from build123d import *

# Parameters (mm, degrees)
BOSS_EXTRUDE1_DEPTH      = 50
FILLET2_R                = 20
SKETCH6_R                = 1.5
CUT_EXTRUDE2_DEPTH       = 28.4
CUT_EXTRUDE3_DEPTH       = 136.4
CUT_EXTRUDE4_DEPTH       = 116.893533958
CUT_EXTRUDE4_DEPTH_BACK  = 26.4
BOSS_EXTRUDE2_DEPTH      = 21.9
BOSS_EXTRUDE3_DEPTH      = 12.1
BOSS_EXTRUDE4_DEPTH      = 7.5
CUT_EXTRUDE5_START       = 12.1
CUT_EXTRUDE5_OUTLINE_R   = 2.25
CUT_EXTRUDE5_DEPTH       = 21.9
CUT_EXTRUDE5_START_2     = -7.5
CUT_EXTRUDE5_2_OUTLINE_R = 4
CUT_EXTRUDE5_2_DEPTH     = 7.5


# Read off the part's stored shape, not the designer's step: Cut-Extrude5
with BuildPart() as part:
    # Sketch1 → Boss-Extrude1 (new body)
    with BuildSketch(Plane(origin=(0, 0, 0), x_dir=(1, 0, 0), z_dir=(0, 1, 0))):
        with BuildLine():
            Line((-56.375697839, 54.197981352), (-56.375697839, 10.497981352))
            ThreePointArc((-56.375697839, 10.497981352), (-53.44676565, 3.42691354), (-46.375697839, 0.497981352))
            Line((-46.375697839, 0.497981352), (16.224302161, 0.497981352))
            ThreePointArc((16.224302161, 0.497981352), (23.295369973, 3.42691354), (26.224302161, 10.497981352))
            Line((26.224302161, 10.497981352), (26.224302161, 64.097981352))
            Line((26.224302161, 64.097981352), (19.224302161, 64.097981352))
            Line((19.224302161, 64.097981352), (19.224302161, 10.497981352))
            ThreePointArc((19.224302161, 10.497981352), (18.345622505, 8.376661008), (16.224302161, 7.497981352))
            Line((16.224302161, 7.497981352), (-46.375697839, 7.497981352))
            ThreePointArc((-46.375697839, 7.497981352), (-48.497018182, 8.376661008), (-49.375697839, 10.497981352))
            Line((-49.375697839, 10.497981352), (-49.375697839, 54.197981352))
            Line((-49.375697839, 54.197981352), (-56.375697839, 54.197981352))
        make_face()
    extrude(amount=BOSS_EXTRUDE1_DEPTH)

    # Fillet2
    fillet2_edges = [part.edges().sort_by_distance(p)[0] for p in [
        (22.724302161, 0, -64.097981352),
        (-52.875697839, 0, -54.197981352),
        (22.724302161, 50, -64.097981352),
        (-52.875697839, 50, -54.197981352),
    ]]
    fillet(fillet2_edges, radius=FILLET2_R)

    # Sketch6 → Cut-Extrude2 (cut)
    with BuildSketch(Plane(origin=(26.224302161, 0, 0), x_dir=(0, 0, -1), z_dir=(1, 0, 0))):
        with BuildLine():
            ThreePointArc((34.097981352, 25), (38.097981352, 21), (42.097981352, 25))
            Line((42.097981352, 25), (34.097981352, 25))
        make_face()
        with BuildLine():
            Line((34.097981352, 25), (42.097981352, 25))
            ThreePointArc((42.097981352, 25), (38.097981352, 29), (34.097981352, 25))
        make_face()
        with BuildLine():
            ThreePointArc((31.836343923, 25), (38.097981352, 18.738362572), (44.35961878, 25))
            Line((44.35961878, 25), (42.097981352, 25))
            ThreePointArc((42.097981352, 25), (38.097981352, 21), (34.097981352, 25))
            Line((34.097981352, 25), (31.836343923, 25))
        make_face()
        with BuildLine():
            Line((42.097981352, 25), (44.35961878, 25))
            ThreePointArc((44.35961878, 25), (38.097981352, 31.261637428), (31.836343923, 25))
            Line((31.836343923, 25), (34.097981352, 25))
            ThreePointArc((34.097981352, 25), (38.097981352, 29), (42.097981352, 25))
        make_face()
        with Locations((30.390517437, 32.707463915)):
            Circle(SKETCH6_R)
        with Locations((26.876196734, 36.221784617)):
            Circle(SKETCH6_R)
        with Locations((23.354804964, 39.743176388)):
            Circle(SKETCH6_R)
        with Locations((19.854626397, 43.243354955)):
            Circle(SKETCH6_R)
        with Locations((44.108388992, 31.01040764)):
            Circle(SKETCH6_R)
        with Locations((47.643922898, 34.545941546)):
            Circle(SKETCH6_R)
        with Locations((51.179456803, 38.081475452)):
            Circle(SKETCH6_R)
        with Locations((54.714990709, 41.617009358)):
            Circle(SKETCH6_R)
        with Locations((45.805445266, 17.292536085)):
            Circle(SKETCH6_R)
        with Locations((49.319765969, 13.778215383)):
            Circle(SKETCH6_R)
        with Locations((52.841157739, 10.256823612)):
            Circle(SKETCH6_R)
        with Locations((56.341336306, 6.756645045)):
            Circle(SKETCH6_R)
        with Locations((32.087573711, 18.98959236)):
            Circle(SKETCH6_R)
        with Locations((28.552039805, 15.454058454)):
            Circle(SKETCH6_R)
        with Locations((25.0165059, 11.918524548)):
            Circle(SKETCH6_R)
        with Locations((21.480971994, 8.382990642)):
            Circle(SKETCH6_R)
    extrude(amount=-CUT_EXTRUDE2_DEPTH, mode=Mode.SUBTRACT)

    # Sketch6<3> → Cut-Extrude3 (cut)
    with BuildSketch(Plane(origin=(26.224302161, 0, 0), x_dir=(0, 0, -1), z_dir=(1, 0, 0))):
        with BuildLine():
            ThreePointArc((34.097981352, 25), (38.097981352, 21), (42.097981352, 25))
            Line((42.097981352, 25), (34.097981352, 25))
        make_face()
        with BuildLine():
            Line((34.097981352, 25), (42.097981352, 25))
            ThreePointArc((42.097981352, 25), (38.097981352, 29), (34.097981352, 25))
        make_face()
    extrude(amount=-CUT_EXTRUDE3_DEPTH, mode=Mode.SUBTRACT)

    # Sketch7 → Cut-Extrude4 (cut, two sides: drawn at the far end of the back side and taken through both)
    with BuildSketch(Plane(origin=(26.224302161, 0, 0), x_dir=(0, 0, -1), z_dir=(1, 0, 0)).offset(-CUT_EXTRUDE4_DEPTH_BACK)):
        with BuildLine():
            Line((44.097981352, 50), (27.901409821, 50))
            Line((27.901409821, 50), (34.889942889, 40.363586132))
            ThreePointArc((34.889942889, 40.363586132), (38.136702541, 38.542544558), (41.629478365, 39.830239282))
            Line((41.629478365, 39.830239282), (48.26230961, 49.561655609))
            ThreePointArc((48.26230961, 49.561655609), (46.191648926, 49.890112018), (44.097981352, 50))
        make_face()
    extrude(amount=CUT_EXTRUDE4_DEPTH + CUT_EXTRUDE4_DEPTH_BACK, mode=Mode.SUBTRACT)

    # Sketch8 → Boss-Extrude2 (add)
    with BuildSketch(Plane(origin=(0, 34, 0), x_dir=(1, 0, 0), z_dir=(0, 1, 0))):
        with BuildLine():
            Line((-52.375697839, 7.497981352), (24.224302161, 7.497981352))
            ThreePointArc((24.224302161, 7.497981352), (27.759836067, 6.033515257), (29.224302161, 2.497981352))
            Line((29.224302161, 2.497981352), (29.224302161, -27.802018648))
            ThreePointArc((29.224302161, -27.802018648), (27.759836067, -31.337552554), (24.224302161, -32.802018648))
            Line((24.224302161, -32.802018648), (19.224302161, -32.802018648))
            Line((19.224302161, -32.802018648), (19.224302161, -2.502018648))
            Line((19.224302161, -2.502018648), (-47.375697839, -2.502018648))
            Line((-47.375697839, -2.502018648), (-47.375697839, -32.802018648))
            Line((-47.375697839, -32.802018648), (-52.375697839, -32.802018648))
            ThreePointArc((-52.375697839, -32.802018648), (-55.911231744, -31.337552554), (-57.375697839, -27.802018648))
            Line((-57.375697839, -27.802018648), (-57.375697839, 2.497981352))
            ThreePointArc((-57.375697839, 2.497981352), (-55.911231744, 6.033515257), (-52.375697839, 7.497981352))
        make_face()
    extrude(amount=-BOSS_EXTRUDE2_DEPTH)

    # Sketch9 → Boss-Extrude3 (add)
    with BuildSketch(Plane.XZ.offset(-12.1)):
        with BuildLine():
            Line((-6.375697839, 2.502018648), (-47.375697839, 2.502018648))
            Line((-47.375697839, 2.502018648), (-57.375697839, 2.502018648))
            Line((-57.375697839, 2.502018648), (-57.375697839, -2.497981352))
            ThreePointArc((-57.375697839, -2.497981352), (-56.882077579, -4.664208864), (-55.498681185, -6.402718861))
            ThreePointArc((-55.498681185, -6.402718861), (-51.809268262, -2.102964231), (-46.375697839, -0.497981352))
            Line((-46.375697839, -0.497981352), (-6.375697839, -0.497981352))
            Line((-6.375697839, -0.497981352), (-6.375697839, 2.502018648))
        make_face()
    extrude(amount=BOSS_EXTRUDE3_DEPTH)

    # Sketch10 → Boss-Extrude4 (add)
    with BuildSketch(Plane.XZ):
        with BuildLine():
            ThreePointArc((-6.375697839, 27.802018648), (-7.840163933, 31.337552554), (-11.375697839, 32.802018648))
            Line((-11.375697839, 32.802018648), (-52.375697839, 32.802018648))
            ThreePointArc((-52.375697839, 32.802018648), (-55.911231744, 31.337552554), (-57.375697839, 27.802018648))
            Line((-57.375697839, 27.802018648), (-57.375697839, -2.497981352))
            ThreePointArc((-57.375697839, -2.497981352), (-55.911231744, -6.033515257), (-52.375697839, -7.497981352))
            Line((-52.375697839, -7.497981352), (-11.375697839, -7.497981352))
            ThreePointArc((-11.375697839, -7.497981352), (-7.840163933, -6.033515257), (-6.375697839, -2.497981352))
            Line((-6.375697839, -2.497981352), (-6.375697839, 27.802018648))
        make_face()
    extrude(amount=BOSS_EXTRUDE4_DEPTH)

    # Cut-Extrude5 outline → Cut-Extrude5 (cut)
    with BuildSketch(Plane(origin=(0, 0, 0), x_dir=(1, 0, 0), z_dir=(0, 1, 0)).offset(CUT_EXTRUDE5_START)):
        with Locations((23.424302161, -26.152018648)):
            Circle(CUT_EXTRUDE5_OUTLINE_R)
        with Locations((23.424302161, -9.152018648)):
            Circle(CUT_EXTRUDE5_OUTLINE_R)
        with Locations((-51.575697839, -9.152018648)):
            Circle(CUT_EXTRUDE5_OUTLINE_R)
        with Locations((-51.575697839, -26.152018648)):
            Circle(CUT_EXTRUDE5_OUTLINE_R)
    extrude(amount=CUT_EXTRUDE5_DEPTH, mode=Mode.SUBTRACT)

    # Cut-Extrude5 2 outline → Cut-Extrude5 2 (cut)
    with BuildSketch(Plane(origin=(0, 0, 0), x_dir=(1, 0, 0), z_dir=(0, 1, 0)).offset(CUT_EXTRUDE5_START_2)):
        with Locations((-33.547970659, -17.65072745)):
            Circle(CUT_EXTRUDE5_2_OUTLINE_R)
    extrude(amount=CUT_EXTRUDE5_2_DEPTH, mode=Mode.SUBTRACT)


solid = part.part
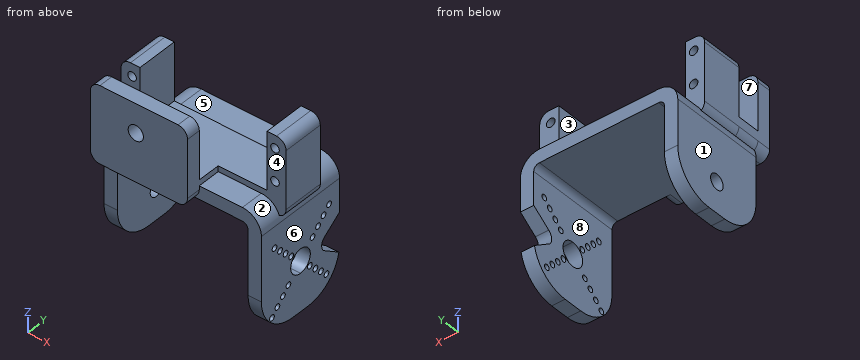
The model under review builds one solid part; all positions refer to its coordinate system, in mm. Face numbers are marked on the shaded views. A direction names the side the tool comes from. Coordinates: 2 decimals unless noted, no trailing zeros. Loops run counter-clockwise (first coordinate to the right, second up) from the corner with the lowest first, then second, coordinate; pieces in that order, holes last. Notation, with made-up numbers: M 34,57.25 L 76,57.25 A31 cw 76,87.25 Z; hole C -15,16 d4. An arc over 180 degrees is marked long. Put each result on its own line as item: value. Start each with the question number.
Q1. Wall thickness on line 1 (X direction, y = 27, z = 9); line 2 (X direction, y = 22, z = -50.5); line 3 (X direction, y = 22, z = 27): over which ranges is each line inside the solid? List them lowest first.
Q2. Add section C-C (x = -17). Write out the cut boundary in (y, z), and give its area (3 significant figures).
Q3. Add section D-D (z = 20.5). Write out the cut boundary in (x, y), and give its area (3 significant figures).
Q4. Add section A-A (z = 4). Write out the cut boundary in (x, y).
Q5. Add section B-B (z = -14.5). Write out the cut boundary in (x, y).
Q6. Clearance check with flat-ended pins moving along their axes: pin 1 (13 mm diameter, centred on y = 23.5, z = -28, fed in from +X); pin 2 (6 mm diameter, centred on x = -40.5, y = 32, fed in from +Z); pin 3 (2 mm diameter, centred on y = 20, z = -48, fed in from -X); pin 4 (6 mm diameter, centred on y = 3.5, z = 10.5, fed in from +X). State where each tip first meets the part, or that it passes through.
Q7. The part is to be moulded in two halves that separate along X. For the marked faces 1, 2 and 3, say which applies: +X half, -X half, draft (parallel to the pull), parting line (faces both ways), or undercut.
Q8. For the marked faces 4, 5, 6, 7 and 8, list the 3-axis set-ups (+Z, -Z, +X, -X, +Y, -Y) from which the entire face can be reached by the end or side of a thin tool; tool diameter is ignored.
Answers:
1. line 1: x = -57.38 to -53.82, -49.33 to -47.38, 19.22 to 21.18, 25.67 to 29.22
1. line 2: x = -56.38 to -49.38, 19.22 to 26.22
1. line 3: x = -57.38 to -53.66, -49.49 to -47.38, 19.22 to 21.34, 25.51 to 29.22
2. outline: M -7.5,-7.5 L 50,-7.5 L 50,-0.5 L 34,-0.5 L 34,2.5 L 0,2.5 L 0,32.8 L -7.5,32.8 Z
2. area: 754 mm^2
3. outline: M -57.38,-7.5 L -36.36,-7.5 L -36.36,0 L -57.38,0 Z; M -57.38,12.1 L -47.38,12.1 L -47.38,34 L -57.38,34 Z; M -30.74,-7.5 L -6.38,-7.5 L -6.38,0 L -30.74,0 Z; M 19.22,12.1 L 29.22,12.1 L 29.22,34 L 19.22,34 Z
3. area: 778 mm^2
4. outline: M -57.38,-7.5 L -6.38,-7.5 L -6.38,0 L -57.38,0 Z; M -57.38,12.1 L -47.38,12.1 L -47.38,34 L -57.38,34 Z; M 19.22,12.1 L 29.22,12.1 L 29.22,34 L 19.22,34 Z
5. outline: M -56.38,0 L -49.38,0 L -49.38,50 L -56.38,50 Z; M 19.22,0 L 26.22,0 L 26.22,50 L 19.22,50 Z
6. pin 1: stops at x = 26.22
6. pin 2: stops at z = 2.5
6. pin 3: stops at x = -56.38
6. pin 4: passes through
7. face 1: -X half
7. face 2: +X half
7. face 3: undercut
8. face 4: +Z, +X, -Y
8. face 5: +Z, +X, -X, +Y
8. face 6: -Z, +X, +Y, -Y
8. face 7: +Z, +X, -X
8. face 8: -Z, +Y, -Y
